The listing builds one solid part. Answer for the finished solid, in the listing's coordinates (mm). Face numbers are marked on the shaded views. A direction names the side the tool comes from. Coordinates: 2 decimals unless noted, no trailing zeros. Order: outer loops, then holes, each group sorted by start corner. A loop starts at its lowest first (then second) coordinate and runs counter-clockwise, first axis right, second up. Notation, with made-up numbers: (61, 65.25) -> (99, 65.25) arc R7 ccw to (99, 69.25) -> close; hole circle Ø7 at (60.25, -33). An arc over 180 degrees is marked (long way). Return JSON: item names as keys, results as strings.
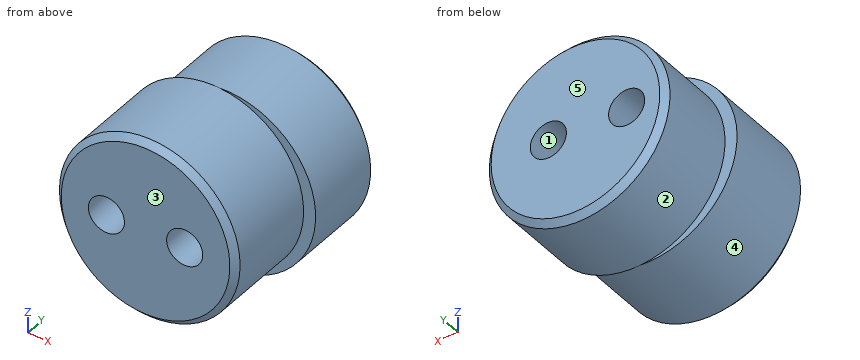
from build123d import *

# Parameters (mm, degrees)
SKETCH1_R           = 7.5
BOSS_EXTRUDE1_DEPTH = 8
SKETCH2_R           = 7.5
BOSS_EXTRUDE2_DEPTH = 7
SKETCH3_R           = 1.5
CUT_EXTRUDE1_DEPTH  = 19.801595677
CHAMFER1_SIZE       = 0.5


with BuildPart() as part:
    # Sketch1 → Boss-Extrude1 (new body)
    with BuildSketch(Plane(origin=(0, 0, 0), x_dir=(1, 0, 0), z_dir=(0, 1, 0))):
        with Locations(Location((0, 0, 0), (0, 0, 270))):
            Circle(SKETCH1_R)
    extrude(amount=BOSS_EXTRUDE1_DEPTH)

    # Sketch2 → Boss-Extrude2 (add)
    with BuildSketch(Plane(origin=(0, 8, 0), x_dir=(1, 0, 0), z_dir=(0, 1, 0))):
        with Locations(Location((1, 0, 0), (0, 0, 93.822553729))):
            Circle(SKETCH2_R)
    extrude(amount=BOSS_EXTRUDE2_DEPTH)

    # Sketch3 → Cut-Extrude1 (cut, through all)
    with BuildSketch(Plane.XZ):
        with Locations(Location((-3.25, 0, 0), (0, 0, 270))):
            Circle(SKETCH3_R)
        with Locations(Location((3.25, 0, 0), (0, 0, 270))):
            Circle(SKETCH3_R)
    extrude(amount=-CUT_EXTRUDE1_DEPTH, mode=Mode.SUBTRACT)

    # Chamfer1
    chamfer1_edges = [part.edges().sort_by_distance(p)[0] for p in [
        (0, 0, -7.5),
        (1.5, 15, 7.483314774),
    ]]
    chamfer(chamfer1_edges, length=CHAMFER1_SIZE)


solid = part.part
1. For the marked faces 4 and 5, determine the directions among +Z, -Z, +X, -X, +Y, -Y from which every point of the face is accessible in a straight line to the end or side of a thin tool.
Answer block:
{"face 4": "-Y", "face 5": "+Z, -Z, +X, -X, +Y"}
2. The part is cut by section A-A on z = 0. Give the vertices of the cut face in (x, y), and give its area (4 significant figures).
Answer block:
{"outline": "(-7.5, 0.5) -> (-7, 0) -> (-4.75, 0) -> (-4.75, 15) -> (-6, 15) -> (-6.5, 14.5) -> (-6.5, 8) -> (-7.5, 8) -> close; (-1.75, 0) -> (1.75, 0) -> (1.75, 15) -> (-1.75, 15) -> close; (4.75, 0) -> (7, 0) -> (7.5, 0.5) -> (7.5, 8) -> (8.5, 8) -> (8.5, 14.5) -> (8, 15) -> (4.75, 15) -> close", "area": "134.5 mm2"}
3. The part is cut by section B-B on y = 2.5. Give the vertices of the cut face in (x, z), and give its area (3 significant figures).
Answer block:
{"outline": "circle Ø15 at (0, 0); hole circle Ø3 at (-3.25, 0); hole circle Ø3 at (3.25, 0)", "area": "163 mm2"}
4. Determine the mould class of the marked faces 1, 2 and 3 for opening direction Z: pulls with the +Z half, pulls with the -Z half, needs draft (parallel to the pull), parting line crosses it, or undercut.
Answer block:
{"face 1": "undercut", "face 2": "parting line crosses it", "face 3": "needs draft"}
5. Consider line 1 (X direction, y = 6, z = 0); line 2 (X direction, y = 9, z = 0); line 3 (Z direction, x = -4.5, y = 7.75). Determine where each line is inside the solid, lowest interval first. Write a range as from..to.
Answer block:
{"line 1": "x = -7.5..-4.75, -1.75..1.75, 4.75..7.5", "line 2": "x = -6.5..-4.75, -1.75..1.75, 4.75..8.5", "line 3": "z = -6..-0.83, 0.83..6"}
6. Each of these flat-tipped pins is pushed along its axis until it touches: pin 1 Ø6 at (y, z) = (4.5, -4) entering from -X; pin 2 Ø1.5 at (x, y) = (-2, 2.5) entering from +Z. Where does it stop, or does it pass through?
Answer block:
{"pin 1": "stops at x = -7.43", "pin 2": "stops at z = 7.4"}
